The listing builds one solid part. Answer for the finished solid, in the listing's coordinates (mm). A direction names the side the tool comes from. Coordinates: 2 decimals unless noted, no trailing zeros. Loops run counter-clockwise (first coordinate to the right, second up) from the corner with the lowest first, then second, coordinate; pieces in that order, holes last. Notation, with made-up numbers: (52.25, 23) - (76.25, 23) arc R23 cw to (76.25, 42) - close; hole circle Ø8 at (11.25, 64). An arc over 180 degrees is marked (long way). One line per question, with ' | ' between items.
from build123d import *

# Parameters (mm, degrees)
F4_DEPTH = 1.5
F3_R     = 1.25
F5_DEPTH = 25
F6_COUNT = 2
F6_ANGLE = 180


with BuildPart() as f1:
    # F0 (on Top) → F1 (revolve)
    with BuildSketch(Plane.XY):
        Polygon((-4.5, 0), (-2.5, 0), (-1.25, 0), (-1.25, 22), (0, 23.25), (0, 26.25), (-4.5, 26.25), (-4.5, 25.25), (-3.75, 25.25), (-3.75, 24.25), (-4.5, 24.25), (-4.5, 20), (-3, 20), (-3, 16.5), (-4.5, 16.5), (-4.5, 11), (-3, 11), (-3, 7.5), (-4.5, 7.5), (-4.5, 2), (-3.75, 2), (-3.75, 1), (-4.5, 1), align=None)
    revolve(axis=Axis((0, 2.3840577891, 0), (0, -1, 0)))

    # F3 (on offset) → F5 (cut)
    with BuildSketch(Plane.XY.offset(4.5)):
        with Locations((0, 14)):
            Circle(F3_R)
        with Locations((0, 18.25)):
            Circle(F3_R)
    extrude(amount=-F5_DEPTH, mode=Mode.SUBTRACT)


with BuildPart() as f4:
    # F3 (on offset) → F4 (new body)
    with BuildSketch(Plane.XY.offset(4.5)):
        with BuildLine():
            Line((-1.25, 8.75), (-1.25, 4.75))
            ThreePointArc((-1.25, 4.75), (0, 3.5), (1.25, 4.75))
            Line((1.25, 4.75), (1.25, 8.75))
            Line((1.25, 8.75), (-1.25, 8.75))
        make_face()
    extrude(amount=-F4_DEPTH)


with BuildPart() as f6_1:
    # F6: instance of F4
    add(f4.part.rotate(Axis((0, 0, 0), (0, -1, 0)), 1 * F6_ANGLE / (F6_COUNT - 1)))


with BuildPart() as f1_1:
    add(f1.part)

    # F7: cut F4, F6_1
    add(f4.part, mode=Mode.SUBTRACT)
    add(f6_1.part, mode=Mode.SUBTRACT)


solid = f1_1.part
Item 1: Find section B-B, the plane x = -3.5. Write down the section's boundary in (y, z), plus the area to 3 significant figures.
Taken from the geometry:
outline: (0, -2.83) - (1, -2.83) - (1, -1.35) - (2, -1.35) - (2, -2.83) - (7.5, -2.83) - (7.5, 2.83) - (2, 2.83) - (2, 1.35) - (1, 1.35) - (1, 2.83) - (0, 2.83) - close; (11, -2.83) - (16.5, -2.83) - (16.5, 2.83) - (11, 2.83) - close; (20, -2.83) - (24.25, -2.83) - (24.25, -1.35) - (25.25, -1.35) - (25.25, -2.83) - (26.25, -2.83) - (26.25, 2.83) - (25.25, 2.83) - (25.25, 1.35) - (24.25, 1.35) - (24.25, 2.83) - (20, 2.83) - close | area: 103 mm2
Item 2: The mould has two halves that part along X. Classify faces 4 (the face through (1, 25.25, -4)), 5 (the face through (0.16, 20.57, -1.24)), 6 (the face through (0.59, 22.1, -4.46)): pulls with the +X half, pulls with the -X half, needs draft (parallel to the pull), parting line crosses it, or undercut.
Taken from the geometry:
face 4: needs draft | face 5: undercut | face 6: parting line crosses it
Item 3: Find the intervals of material crossed by line 1 (Y direction, x = 0, z = -3.1); line 2 (Y direction, x = 0, z = -1.95); line 3 (Y direction, x = 3.5, z = 1.5), in increasing order. Write a range as [from, to].
Taken from the geometry:
line 1: y = [0, 3.5], [11, 12.75], [15.25, 16.5], [20, 26.25] | line 2: y = [0, 12.75], [15.25, 17], [19.5, 26.25] | line 3: y = [0, 1], [2, 7.5], [11, 16.5], [20, 24.25], [25.25, 26.25]
Item 4: Find section A-A, the plane z = -3.5. State how many separate pieces and enclosed holes the cut face has, plus the area to 3 significant figures.
Taken from the geometry:
separate pieces: 3 | enclosed holes: 1 | area: 88.7 mm2
Item 5: Each of these flat-tipped pins is pushed along its axis until it touches: pin 1 Ø1 at (x, y) = (1, 16.5) entering from -Z; pin 2 Ø1.2 at (x, y) = (0, 6.5) entering from -Z; pin 3 Ø3 at (y, z) = (13, -2.5) entering from +X. Where does it stop, or does it pass through?
Taken from the geometry:
pin 1: stops at z = -4.47 | pin 2: stops at z = -3 | pin 3: stops at x = 4.39
Item 6: Which of the six approach directions +Z, -Z, +X, -X, +Y, -Y give full straight-line access (tool end or side, diameter ignored) to faces 1 (the face through (0, 3.5, -3.8)), 2 (the face through (-1, 1, -4)), 3 (the face through (3.2, 7.5, -0.1))?
Taken from the geometry:
face 1: -Z | face 2: none | face 3: +X
Item 7: Find section C-C, the plane y = 14.25. Write down the section's boundary in (x, z), plus the area to 3 significant figures.
Taken from the geometry:
outline: (-1.22, -4.33) - (-1.22, -0.25) arc R1.25 cw to (-1.22, 0.25) - (-1.22, 4.33) arc R4.5 ccw to start; (1.22, -4.33) arc R4.5 ccw to (1.22, 4.33) - (1.22, 0.25) arc R1.25 cw to (1.22, -0.25) - close | area: 41.8 mm2
